Geometry: see drawing. Coordinates: mm, zero at the bounding-box minimum. Give positions to 0.01 mm unless a question says otherwise; leave off trailing zeros. Write each loop counter-clockwise with the first axis right and the second up, starting at its lowest first coordinate (ties: lowest second). Pieces come first, ordered by that corner, then holes. Notation, with made-up numbers: (65.25, -6) -> (103.25, -6) arc R16 ccw to (103.25, 17) -> close; hole circle Ø11 at (44.25, 51.25). An arc over 180 degrees is marked (long way). Use one line per item in the form item = value. Start each with the question number.
(1) Cut plane A-A, the plane x = 142.5. Output: boundary loops of the cut face in (y, z), and give its area (3 significant figures).
(2) Cut plane B-B, the plane y = 11. Output: boundary loops of the cut face in (x, z).
(3) Material intervals for line 1 along Y through (x, z) = (182.5, 1.25); line 2 along Y through (x, z) = (142.5, 1.35); line 3 along X through (y, z) = (37, 0.35), sorted ascending. Write a range as from..to.
(4) Draft query along Z for the marked faces 1 and 2. Return one class per face: pulls with the +Z half, pulls with the -Z half, needs draft (parallel to the pull), parting line crosses it, or undercut.
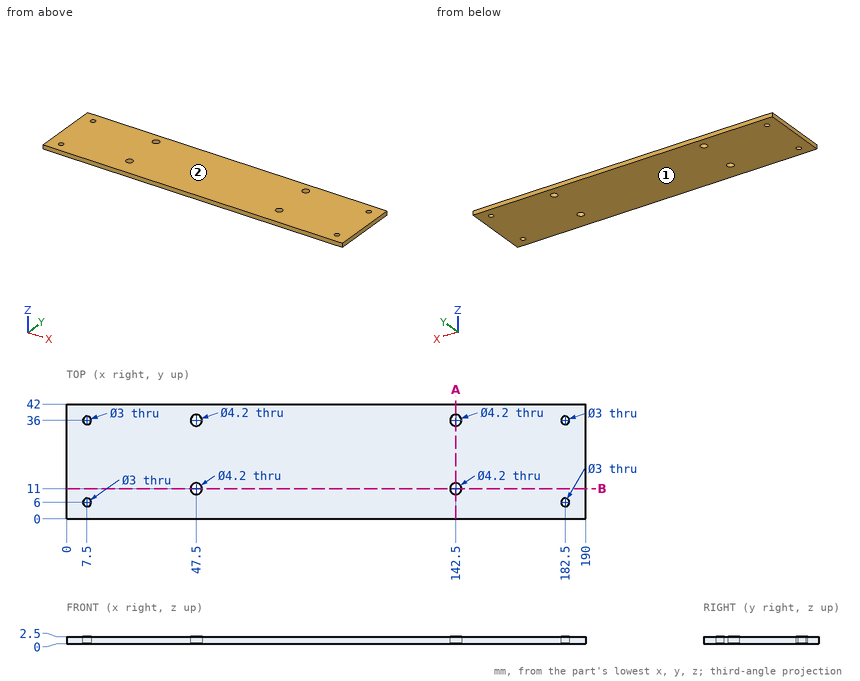
Geometry says:
q1.outline = (0, 0) -> (8.9, 0) -> (8.9, 2.5) -> (0, 2.5) -> close; (13.1, 0) -> (33.9, 0) -> (33.9, 2.5) -> (13.1, 2.5) -> close; (38.1, 0) -> (42, 0) -> (42, 2.5) -> (38.1, 2.5) -> close
q1.area = 84.0 mm^2
q2.outline = (0, 0) -> (45.4, 0) -> (45.4, 2.5) -> (0, 2.5) -> close; (49.6, 0) -> (140.4, 0) -> (140.4, 2.5) -> (49.6, 2.5) -> close; (144.6, 0) -> (190, 0) -> (190, 2.5) -> (144.6, 2.5) -> close
q3.line_1 = 0..4.5, 7.5..34.5, 37.5..42
q3.line_2 = 0..8.9, 13.1..33.9, 38.1..42
q3.line_3 = 0..6.38, 8.62..45.65, 49.35..140.65, 144.35..181.38, 183.62..190
q4.face_1 = pulls with the -Z half
q4.face_2 = pulls with the +Z half
